from build123d import *

# Parameters (mm, degrees)
SKIZZE1_R                       = 4.57
SKIZZE1_R_2                     = 2
AUFSATZ_LINEAR_AUSTRAGEN1_DEPTH = 13
SCHNITT_LINEAR_AUSTRAGEN1_DEPTH = 14
VERRUNDUNG1_R                   = 0.5
KREISMUSTER1_COUNT              = 10
VERRUNDUNG1_OF_KREISMUSTER1_R   = 0.5
FASE2_SIZE                      = 0.2
BOSS_EXTRUDE1_DEPTH             = 6.3
BOSS_EXTRUDE1_DEPTH_BACK        = 6.3
SKETCH2_R                       = 2.2
BOSS_EXTRUDE4_DEPTH             = 13
SKETCH3_R                       = 2
BOSS_EXTRUDE6_DEPTH             = 5
BOSS_EXTRUDE6_DEPTH_BACK        = 15.5
FILLET2_R                       = 0.5
SKETCH4_R                       = 2.5
SKETCH4_R_2                     = 1.5
BOSS_EXTRUDE7_DEPTH             = 1.5
FILLET3_R                       = 0.25
SKETCH5_R                       = 2.5
SKETCH5_R_2                     = 1.5
BOSS_EXTRUDE8_DEPTH             = 4
FILLET4_R                       = 0.5


with BuildPart() as part:
    # Skizze1 → Aufsatz-Linear austragen1 (new body)
    with BuildSketch(Plane(origin=(0, 0, 0), x_dir=(1, 0, 0), z_dir=(0, 1, 0))):
        Circle(SKIZZE1_R)
        Circle(SKIZZE1_R_2, mode=Mode.SUBTRACT)
    extrude(amount=AUFSATZ_LINEAR_AUSTRAGEN1_DEPTH)

    # Skizze12 → Schnitt-Linear austragen1 (cut, through all)
    with BuildSketch(Plane(origin=(0, 13, 0), x_dir=(1, 0, 0), z_dir=(0, 1, 0))):
        with BuildLine():
            Line((-1.2, 4.409637173), (-0.808470756, 3.57))
            Line((-0.808470756, 3.57), (0.808470756, 3.57))
            Line((0.808470756, 3.57), (1.2, 4.409637173))
            ThreePointArc((1.2, 4.409637173), (0, 4.57), (-1.2, 4.409637173))
        make_face()
    schnitt_linear_austragen1 = extrude(amount=-SCHNITT_LINEAR_AUSTRAGEN1_DEPTH, mode=Mode.SUBTRACT)

    # Verrundung1
    verrundung1_edges = [part.edges().sort_by_distance(p)[0] for p in [
        (0.808470756, 6.5, -3.57),
        (-0.808470756, 6.5, -3.57),
    ]]
    fillet(verrundung1_edges, radius=VERRUNDUNG1_R)

    # Kreismuster1: Schnitt-Linear austragen1 ×10 about axis
    kreismuster1_axis = Axis((0, 0, 0), (0, 1, 0))
    for i in range(1, KREISMUSTER1_COUNT):
        add(schnitt_linear_austragen1.rotate(kreismuster1_axis, i * 360 / KREISMUSTER1_COUNT), mode=Mode.SUBTRACT)

    # Verrundung1 of Kreismuster1
    verrundung1_of_kreismuster1_edges = [part.edges().sort_by_distance(p)[0] for p in [
        (-1.44432677, 6.5, -3.363397857),
        (-2.752459932, 6.5, -2.412983483),
        (-3.14544056, 6.5, -1.872092051),
        (-3.645102966, 6.5, -0.334289289),
        (-3.645102966, 6.5, 0.334289289),
        (-3.14544056, 6.5, 1.872092051),
        (-2.752459932, 6.5, 2.412983483),
        (-1.44432677, 6.5, 3.363397857),
        (-0.808470756, 6.5, 3.57),
        (0.808470756, 6.5, 3.57),
        (1.44432677, 6.5, 3.363397857),
        (2.752459932, 6.5, 2.412983483),
        (3.14544056, 6.5, 1.872092051),
        (3.645102966, 6.5, 0.334289289),
        (3.645102966, 6.5, -0.334289289),
        (3.14544056, 6.5, -1.872092051),
        (2.752459932, 6.5, -2.412983483),
        (1.44432677, 6.5, -3.363397857),
    ]]
    fillet(verrundung1_of_kreismuster1_edges, radius=VERRUNDUNG1_OF_KREISMUSTER1_R)

    # Fase2
    fase2_edges = [part.edges().sort_by_distance(p)[0] for p in [
        (-2, 0, 0),
        (-2, 13, 0),
    ]]
    chamfer(fase2_edges, length=FASE2_SIZE)

    # Sketch1 → Boss-Extrude1 (add, two sides)
    with BuildSketch(Plane(origin=(0, 6.5, 0), x_dir=(-1, 0, 0), z_dir=(0, -1, 0))) as boss_extrude1_sk:
        with BuildLine():
            Line((-1.4, 1.428285686), (-1.4, -1.428285686))
            ThreePointArc((-1.4, -1.428285686), (-2, 0), (-1.4, 1.428285686))
        make_face()
    extrude(amount=BOSS_EXTRUDE1_DEPTH)
    extrude(boss_extrude1_sk.sketch, amount=-BOSS_EXTRUDE1_DEPTH_BACK)



with BuildPart() as body_2:
    # Sketch2 → Boss-Extrude4 (new body)
    with BuildSketch(Plane(origin=(0, 13, 0), x_dir=(1, 0, 0), z_dir=(0, 1, 0))):
        Circle(SKETCH2_R)
    extrude(amount=-BOSS_EXTRUDE4_DEPTH)


with BuildPart() as part_1:
    add(part.part)

    add(body_2.part)  # Boss-Extrude6 merges body 2
    # Sketch3 → Boss-Extrude6 (add, two sides)
    with BuildSketch(Plane(origin=(0, 13, 0), x_dir=(1, 0, 0), z_dir=(0, 1, 0))) as boss_extrude6_sk:
        Circle(SKETCH3_R)
    extrude(amount=BOSS_EXTRUDE6_DEPTH)
    extrude(boss_extrude6_sk.sketch, amount=-BOSS_EXTRUDE6_DEPTH_BACK)

    # Fillet2
    fillet2_edges = [part_1.edges().sort_by_distance(p)[0] for p in [
        (-2, 13, 0),
        (-2, 0, 0),
    ]]
    fillet(fillet2_edges, radius=FILLET2_R)

    # Sketch4 → Boss-Extrude7 (add)
    with BuildSketch(Plane.XZ):
        Circle(SKETCH4_R)
        Circle(SKETCH4_R_2, mode=Mode.SUBTRACT)
    extrude(amount=BOSS_EXTRUDE7_DEPTH)

    # Fillet3
    fillet3_edges = [part_1.edges().sort_by_distance(p)[0] for p in [
        (-2.5, 0, 0),
    ]]
    fillet(fillet3_edges, radius=FILLET3_R)

    # Sketch5 → Boss-Extrude8 (add)
    with BuildSketch(Plane(origin=(0, 13, 0), x_dir=(1, 0, 0), z_dir=(0, 1, 0))):
        Circle(SKETCH5_R)
        Circle(SKETCH5_R_2, mode=Mode.SUBTRACT)
    extrude(amount=BOSS_EXTRUDE8_DEPTH)

    # Fillet4
    fillet4_edges = [part_1.edges().sort_by_distance(p)[0] for p in [
        (-2.5, 13, 0),
    ]]
    fillet(fillet4_edges, radius=FILLET4_R)


solid = part_1.part
Model file for the job. Use its own axes, mm. A direction names the side the tool comes from. Round coordinates to 2 decimals unless told otherwise and drop trailing zeros. Loops run counter-clockwise (first coordinate to the right, second up) from the corner with the lowest first, then second, coordinate; pieces in that order, holes last. Notation, with made-up numbers: M 34.25,62.25 L 63.25,62.25 A21 cw 63.25,93.25 Z; hole C 59.5,-15 d6. An arc over 180 degrees is marked long. One line per question, with ' | ' between items.
1) Band-saw the part on D-D (x = 4.25). Give the cut face in (y, z), then the cut area to 3 significant figures.
Solved:
outline: M 0,-0.26 L 13,-0.26 L 13,0.26 L 0,0.26 Z | area: 6.76 mm²
2) Band-saw the part on C-C (y = 14). Give the cut face in (x, z), then the cut area to 3 significant figures.
Solved:
outline: C 0,0 d5 | area: 19.6 mm²
3) Mould opens along Z. For faces 1 (the cylindrical face through (0, -2, 2)), 2 (the flat face through (0, -2.5, 0)), 3 (the flat face through (3.393, 6.591, -1.11)) say: +Z half, -Z half, draft (parallel to the pull), parting line (faces both ways), or undercut.
Solved:
face 1: parting line | face 2: draft | face 3: undercut
4) Band-saw the part on B-B (z = 0). Give the cut face in (x, y).
Solved:
outline: M -4.57,0 L -2.75,0 A0.25 cw -2.5,-0.25 L -2.5,-1.5 L -2,-1.5 L -2,-2.5 L 2,-2.5 L 2,-1.5 L 2.5,-1.5 L 2.5,-0.25 A0.25 cw 2.75,0 L 4.57,0 L 4.57,13 L 3,13 A0.5 cw 2.5,13.5 L 2.5,17 L 2,17 L 2,18 L -2,18 L -2,17 L -2.5,17 L -2.5,13.5 A0.5 cw -3,13 L -4.57,13 Z
5) Band-saw the part on A-A (x = 0). Give the cut face in (y, z), then the cut area to 3 significant figures.
Solved:
outline: M -2.5,-2 L -1.5,-2 L -1.5,-2.5 L -0.25,-2.5 A0.25 cw 0,-2.75 L 0,-3.57 L 13,-3.57 L 13,-3 A0.5 cw 13.5,-2.5 L 17,-2.5 L 17,-2 L 18,-2 L 18,2 L 17,2 L 17,2.5 L 13.5,2.5 A0.5 cw 13,3 L 13,3.57 L 0,3.57 L 0,2.75 A0.25 cw -0.25,2.5 L -1.5,2.5 L -1.5,2 L -2.5,2 Z | area: 128 mm²
6) 3-axis set-ups, long thin cutter, end or side, ignore diameter. For faces 4 (the cylindrical face through (-0.54, 15.23, 2.44)), 5 (the flat face through (-1, -1.5, 2)), 6 (the flat face through (-3.397, 6.591, -1.097)): which of +Z, -Z, +X, -X, +Y, -Y reach the whole face in a straight line?
Solved:
face 4: +Y | face 5: -Y | face 6: -X, +Y, -Y
7) Flat gauge pins, fed straight in: pin 1 (0.5 mm diameter, centred on x = 0, y = 6, fed in from +Z); pin 2 (4 mm diameter, centred on x = -2.5, y = 9.5, fed in from -Z); pin 3 (0.5 mm diameter, centred on x = 0, y = 6, fed in from -Z). Where does each tip first touch, or does it go through?
Solved:
pin 1: stops at z = 3.57 | pin 2: stops at z = -4.41 | pin 3: stops at z = -3.57
8) Drill centre lines: line 1 along Z through (x, y) = (3.75, 4); line 2 along X through (y, z) = (2.25, -1.75); line 3 along Y through (x, z) = (1.25, -3). Where is each one in solid material? Low to high.
Solved:
line 1: z = -2.61 to -2.44, -0.37 to 0.37, 2.44 to 2.61 | line 2: x = -3.22 to 3.22 | line 3: y = 0 to 13
